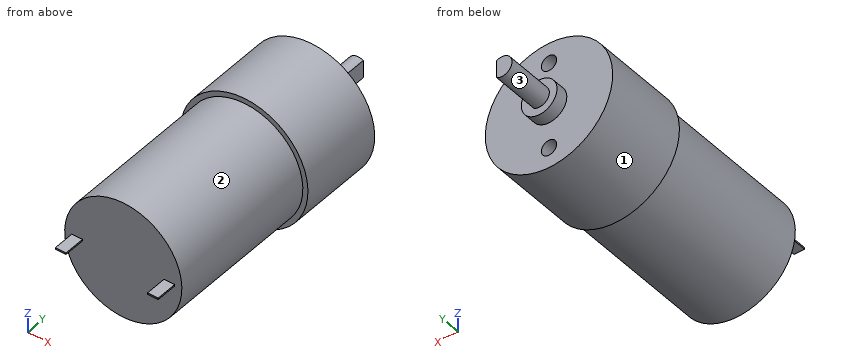
from build123d import *

# Parameters (mm, degrees)
SKETCH2_R           = 12.5
SKETCH2_R_2         = 2
SKETCH2_R_3         = 3.5
BOSS_EXTRUDE1_DEPTH = 17
SKETCH2_3_R         = 2
BOSS_EXTRUDE2_DEPTH = 12
SKETCH2_4_R         = 3.5
SKETCH2_4_R_2       = 2
BOSS_EXTRUDE3_DEPTH = 2.5
SKETCH4_R           = 11.5
BOSS_EXTRUDE4_DEPTH = 30.8
SKETCH5_W           = 2.1
SKETCH5_H           = 0.3
BOSS_EXTRUDE5_DEPTH = 4.2
SKETCH6_R           = 1.5
CUT_EXTRUDE1_DEPTH  = 5
CUT_EXTRUDE2_START  = -9.5
CUT_EXTRUDE2_DEPTH  = 9.5


with BuildPart() as part:
    # Sketch2 → Boss-Extrude1 (new body)
    # profile 1 of 3: a face of its own
    with BuildSketch(Plane(origin=(0, 0, 0), x_dir=(1, 0, 0), z_dir=(0, 1, 0))):
        with Locations(Location((0, 0, 0), (0, 0, 270))):
            Circle(SKETCH2_R)
        Circle(SKETCH2_R_2, mode=Mode.SUBTRACT)
    # profile 2 of 3: a face of its own
    with BuildSketch(Plane(origin=(0, 0, 0), x_dir=(1, 0, 0), z_dir=(0, 1, 0))):
        Circle(SKETCH2_R_3)
        Circle(SKETCH2_R_2, mode=Mode.SUBTRACT)
    # profile 3 of 3: a face of its own
    with BuildSketch(Plane(origin=(0, 0, 0), x_dir=(1, 0, 0), z_dir=(0, 1, 0))):
        Circle(SKETCH2_R_2)
    extrude(amount=-BOSS_EXTRUDE1_DEPTH)

    # Sketch2<3> → Boss-Extrude2 (add)
    with BuildSketch(Plane(origin=(0, 0, 0), x_dir=(1, 0, 0), z_dir=(0, 1, 0))):
        with Locations(Location((0, 0, 0), (0, 0, 270))):
            Circle(SKETCH2_3_R)
    extrude(amount=BOSS_EXTRUDE2_DEPTH)

    # Sketch2<4> → Boss-Extrude3 (add)
    with BuildSketch(Plane(origin=(0, 0, 0), x_dir=(1, 0, 0), z_dir=(0, 1, 0))):
        with Locations(Location((0, 0, 0), (0, 0, 270))):
            Circle(SKETCH2_4_R)
        with Locations(Location((0, 0, 0), (0, 0, 270))):
            Circle(SKETCH2_4_R_2, mode=Mode.SUBTRACT)
    extrude(amount=BOSS_EXTRUDE3_DEPTH)

    # Sketch4 → Boss-Extrude4 (add)
    with BuildSketch(Plane.XZ.offset(17)):
        with Locations(Location((0, 0, 0), (0, 0, 90))):
            Circle(SKETCH4_R)
    extrude(amount=BOSS_EXTRUDE4_DEPTH)

    # Sketch5 → Boss-Extrude5 (add)
    with BuildSketch(Plane.XZ.offset(47.8)):
        with Locations((-9.05, 0)):
            Rectangle(SKETCH5_W, SKETCH5_H)
        with Locations((9.05, 0)):
            Rectangle(SKETCH5_W, SKETCH5_H)
    extrude(amount=BOSS_EXTRUDE5_DEPTH)

    # Sketch6 → Cut-Extrude1 (cut)
    with BuildSketch(Plane(origin=(0, 0, 0), x_dir=(1, 0, 0), z_dir=(0, 1, 0))):
        with Locations(Location((0, -8.5, 0), (0, 0, 270))):
            Circle(SKETCH6_R)
        with Locations(Location((0, 8.5, 0), (0, 0, 90))):
            Circle(SKETCH6_R)
    extrude(amount=-CUT_EXTRUDE1_DEPTH, mode=Mode.SUBTRACT)

    # Sketch7 → Cut-Extrude2 (cut)
    with BuildSketch(Plane(origin=(0, 12, 0), x_dir=(1, 0, 0), z_dir=(0, 1, 0)).offset(CUT_EXTRUDE2_START)):
        with BuildLine():
            ThreePointArc((1, -1.732050808), (2, 0), (1, 1.732050808))
            Line((1, 1.732050808), (1, -1.732050808))
        make_face()
    extrude(amount=CUT_EXTRUDE2_DEPTH, mode=Mode.SUBTRACT)


solid = part.part
Here's how the part is built. I have some questions about the finished solid (model axes, mm). Face numbers are marked on the shaded views. A direction names the side the tool comes from. Coordinates: 2 decimals unless noted, no trailing zeros. Loops run counter-clockwise (first coordinate to the right, second up) from the corner with the lowest first, then second, coordinate; pieces in that order, holes last.
1. Imagine slicing it at B-B, the plane z = -8.5. Please give me the cut outline in (x, y), and give its area (3 significant figures).
2. I need wall thicknesses on L1, parallel to X at y = -18, z = 5.5; L2, parallel to Y at x = -5, z = -1.25; L3, parallel to X at y = -2.95, z = 8.5. Which ranges of each line are inside material? Lowest first, please.
3. Imagine slicing it at A-A, the plane x = 0. Please give me the cut outline in (y, z).
4. For P1, Ø11.5, axis at x = 0, z = 4.5, coming from the -Y side; P2, Ø1, axis at y = 9.5, z = 0, coming from the +X side; P3, Ø1, axis at x = -2, y = -25.5, coming from the +Z side; P4, Ø12, axis at y = -9, z = 4, coming from the -X side, each with a flat end and sliding along its axis, tell me the tip position at first contact or that it passes through.
5. Imagine slicing it at C-C, the plane y = -18.5. Please give me the cut outline in (x, z).
6. For the marked faces 1, 2 and 3, which set-ups out of +Z, -Z, +X, -X, +Y, -Y let a thin tool reach every point of the face, with its end or its side?
7. Imagine slicing it at D-D, the plane x = -5.5. Please give me the cut outline in (y, z).
Taken from the geometry:
1. outline: (-9.17, -17) - (-7.75, -17) - (-7.75, -47.8) - (7.75, -47.8) - (7.75, -17) - (9.17, -17) - (9.17, 0) - (1.5, 0) - (1.5, -5) - (-1.5, -5) - (-1.5, 0) - (-9.17, 0) - close
1. area: 774 mm2
2. L1: x = -10.1 to 10.1
2. L2: y = -47.8 to 0
2. L3: x = -9.17 to -1.5, 1.5 to 9.17
3. outline: (-47.8, -11.5) - (-17, -11.5) - (-17, -12.5) - (0, -12.5) - (0, -10) - (-5, -10) - (-5, -7) - (0, -7) - (0, -3.5) - (2.5, -3.5) - (2.5, -2) - (12, -2) - (12, 2) - (2.5, 2) - (2.5, 3.5) - (0, 3.5) - (0, 7) - (-5, 7) - (-5, 10) - (0, 10) - (0, 12.5) - (-17, 12.5) - (-17, 11.5) - (-47.8, 11.5) - close
4. P1: stops at y = -47.8
4. P2: stops at x = 1
4. P3: stops at z = 11.4
4. P4: stops at x = -12.5
5. outline: circle Ø23 at (0, 0)
6. face 1: +Y, -Y
6. face 2: -Y
6. face 3: +Y
7. outline: (-47.8, -10.1) - (-17, -10.1) - (-17, -11.22) - (0, -11.22) - (0, 11.22) - (-17, 11.22) - (-17, 10.1) - (-47.8, 10.1) - close
